Autodesk Inventor part; units mm, degrees
ref_plane "YZ Plane" through (0, 0, 0) normal (1, 0, 0) x (0, 1, 0)
ref_plane "XZ Plane" through (0, 0, 0) normal (0, 1, 0) x (-1, 0, 0)
ref_plane "XY Plane" through (0, 0, 0) normal (0, 0, 1) x (1, 0, 0)
sketch "Sketch1" plane through (0, 0, 0) normal (0, 1, 0) x (-1, 0, 0)
  line L0 (0, 0) -> (279.4, 0)
  line L1 (279.4, 0) -> (279.4, -50.8)
  line L2 (279.4, -50.8) -> (0, -50.8)
  line L3 (0, -50.8) -> (0, 0)
  dimension "d0" = 279.4
  dimension "d1" = 50.8
extrude "Extrusion1" add sketch "Sketch1" along normal blind 3.175
sketch "Sketch2" plane through (0, 3.175, 0) normal (0, 1, 0) x (1, 0, 0)
  line L0 (-279.4, 0) -> (0, 0)
  line L1 (-279.4, 0) -> (0, 0)
  line L2 (0, 0) -> (0, 3.175)
  line L3 (0, 3.175) -> (-279.4, 3.175)
  line L4 (-279.4, 3.175) -> (-279.4, 0)
  dimension "d4" = 279.4
  dimension "d5" = 3.175
extrude "Extrusion2" add sketch "Sketch2" along normal blind 25.4
sketch "Sketch3" plane through (0, 3.175, 0) normal (0, 1, 0) x (1, 0, 0)
  line L0 (0, 3.175) -> (0, 50.8) construction
  line L1 (0, 50.8) -> (-279.4, 50.8) construction
  line L2 (-139.7, 50.8) -> (-139.7, 9.398) construction
  line L3 (-279.4, 50.8) -> (-248.5898, 50.8) construction
  line L4 (-248.5898, 50.8) -> (-248.5898, 26.797) construction
  circle A0 centre (-248.5898, 26.797) radius 2.5797
  line L5 (-248.5898, 26.797) -> (-264.1372, 37.8052) construction
  circle A1 centre (-264.1372, 37.8052) radius 2.5797
  point P0 (0, 0)
extrude "Extrusion3" cut sketch "Sketch3" against normal blind 25.4
sketch "Sketch4" plane through (0, 3.175, 0) normal (0, 1, 0) x (1, 0, 0)
  line L0 (0, 3.175) -> (0, 50.8) construction
  line L1 (0, 50.8) -> (-279.4, 50.8) construction
  line L2 (0, 23.1034) -> (-12.7, 23.1034) construction
  line L3 (-12.7, 50.8) -> (-12.7, 28.575) construction
  circle A0 centre (-12.7, 28.575) radius 2.5797
  point P0 (0, 0)
  dimension "d26" = 12.7
  dimension "d27" = 22.225
  dimension "d28" = 5.1594
extrude "Extrusion4" cut sketch "Sketch4" against normal blind 25.4
properties part number "angle iron with  holes 2"
Could you check a few things on this model? Use its own coordinates, in mm. A direction names the side the tool comes from. Give positions to 0.01 mm unless a question says otherwise; leave off trailing zeros. Order: outer loops, then holes, each group sorted by start corner. A loop starts at its lowest first (then second) coordinate and runs counter-clockwise, first axis right, second up.
Item 1: I'm going to push flat-ended pins straight in: pin 1 (8.5 mm diameter, centred on x = -264.14, z = -37.81, fed in from +Y) (3 decimals); pin 2 (6 mm diameter, centred on y = 8, z = -34.5, fed in from -X). Where does each tip first touch, or does it pass through?
Item 2: If we section it at B-B, the plane y = 22.75: Write out the boundary of the cut face in (x, z) (3 decimals), plus the area to 3 significant figures.
Item 3: For faces 1 (the face through (-138, 0, -25)), 2 (the face through (-138, 16, -3.175)), which set-ups out of +Z, -Z, +X, -X, +Y, -Y let a thin tool reach every point of the face, with its end or its side?
Item 4: I need wall thicknesses on line 1 (Z direction, x = -12.7, y = 1.2); line 2 (Z direction, x = -104, y = 4.5) (3 decimals); line 3 (Y direction, x = -21, z = -4.5) (3 decimals). Which ranges of each line are inside material? Lowest first, please.
Item 5: If we mould it in two halves opening along Z, with no side actions, what happens to faces 3 (the face through (-266.714, 1.61, -37.919)), 4 (the face through (-138, 14, 0)), 5 (the face through (-138, 3.175, -27)), 6 (the face through (-251.167, 1.61, -26.91))? For each: pulls with the +Z half, pulls with the -Z half, needs draft (parallel to the pull), parting line crosses it, or undercut.
Item 6: If we section it at A-A, the plane x = -12.7: Write out the boundary of the cut face in (y, z) (3 decimals).
Values:
1. pin 1: stops at y = 3.175
1. pin 2: passes through
2. outline: (-279.4, -3.175) - (0, -3.175) - (0, 0) - (-279.4, 0) - close
2. area: 887 mm2
3. face 1: +Z, -Z, +X, -X, -Y
3. face 2: -Z, +X, -X, +Y
4. line 1: z = -50.8 to -31.15, -26 to 0
4. line 2: z = -3.175 to 0
4. line 3: y = 0 to 3.175
5. face 3: undercut
5. face 4: pulls with the +Z half
5. face 5: needs draft
5. face 6: undercut
6. outline: (0, -50.8) - (3.175, -50.8) - (3.175, -31.155) - (0, -31.155) - close; (0, -25.995) - (3.175, -25.995) - (3.175, -3.175) - (28.575, -3.175) - (28.575, 0) - (0, 0) - close
